from build123d import *

# Parameters (mm, degrees)
F0_W     = 36.068
F0_H     = 9.5504
F0_R     = 1.524
F0_H_2   = 16.9672
F0_W_2   = 16.002
F0_R_2   = 2.2225
F1_DEPTH = 1.7018
F2_R     = 2.54
F3_R     = 2.54
F4_W     = 5.766904
F4_H     = 5.702107
F5_DEPTH = 1.778


with BuildPart() as f1:
    # F0 (on Top) → F1 (new body)
    with BuildSketch(Plane.XY):
        with Locations((0, -13.2588)):
            Rectangle(F0_W, F0_H)
        with Locations((-15.167683, -15.197962)):
            Circle(F0_R, mode=Mode.SUBTRACT)
        with Locations((15.185317, -15.197962)):
            Circle(F0_R, mode=Mode.SUBTRACT)
        Rectangle(F0_W, F0_H_2)
        with Locations((-26.035, 0)):
            Rectangle(F0_W_2, F0_H_2)
        with Locations((-29.552327, -3.693333)):
            Circle(F0_R_2, mode=Mode.SUBTRACT)
        with Locations((-29.552327, 3.545667)):
            Circle(F0_R_2, mode=Mode.SUBTRACT)
        with Locations((0, 13.2588)):
            Rectangle(F0_W, F0_H)
        with Locations((-15.167683, 15.155038)):
            Circle(F0_R, mode=Mode.SUBTRACT)
        with Locations((15.185317, 15.155038)):
            Circle(F0_R, mode=Mode.SUBTRACT)
    extrude(amount=F1_DEPTH)

    # F2
    f2_edges = [f1.edges().sort_by_distance(p)[0] for p in [
        (-18.034, 18.034, 0.8509),
        (-18.034, -18.034, 0.8509),
        (18.034, -18.034, 0.8509),
        (18.034, 18.034, 0.8509),
    ]]
    fillet(f2_edges, radius=F2_R)

    # F3
    f3_edges = [f1.edges().sort_by_distance(p)[0] for p in [
        (-18.034, 8.4836, 0.8509),
        (-18.034, -8.4836, 0.8509),
        (-34.036, -8.4836, 0.8509),
        (-34.036, 8.4836, 0.8509),
    ]]
    fillet(f3_edges, radius=F3_R)

    # F4 (on face) → F5 (join)
    with BuildSketch(Plane.XY.offset(1.7018)):
        with Locations((-4.934564, 7.768857)):
            Rectangle(F4_W, F4_H)
    extrude(amount=F5_DEPTH)


solid = f1.part
Read the model definition and answer for the solid it produces. Units are mm, in the model's axes. A direction names the side the tool comes from. Give positions to 0.01 mm unless a question says otherwise; leave off trailing zeros. Write each loop counter-clockwise with the first axis right and the second up, starting at its lowest first coordinate (ties: lowest second). Pieces come first, ordered by that corner, then holes. Notation, with made-up numbers: M 66.25,29 L 102.25,29 A20 cw 102.25,51 Z; hole C -37,10 d6. An arc over 180 degrees is marked long. One line per item, written item: value. Start each with the question number.
(1) Find section A-A (x = -3). Determine the outline of the cut face in (y, z).
(2) Find section D-D (z = 1.1). Determine the outline of the cut face in (x, y) (1 decimal), plus the area to 3 significant figures.
(3) Flat-ended cylindrical pins translate along their axes: pin 1 Ø5 at (x, y) = (-9.5, 11) entering from -Z; pin 2 Ø0.5 at (y, z) = (7.5, 2.5) entering from +X; pin 3 Ø1.4 at (y, z) = (14, 0.5) entering from -X; pin 4 Ø2.5 at (x, y) = (15.19, 15.16) entering from +Z. Find the tip coordinate at first contact, or state that the pin passes through.
(4) A tool of negligible diameter and unlimited length cuts with its end or side. For faces 4 (the cylindrical face through (-27.43, -3.03, 0.84)), 5 (the flat face through (-2.051, 8, 3)), 6 (the flat face through (-5, 10.62, 3)), 7 (the flat face through (-18.034, 13, 1)), 8 (the flat face through (-18.034, -13, 1)), from which of +Z, -Z, +X, -X, +Y, -Y can it reach the whole face along a straight path? Write none if from no direction.
(5) Find section C-C (x = -14.5). Determine the outline of the cut face in (y, z) (3 decimals), plus the area to 3 significant figures.
(6) Find the intervals of material crossed by line 1 (X direction, y = -14, z = 1.25); line 2 (X direction, y = 16, z = 1.3); line 3 (Z direction, x = 7, y = -16), in increasing order.
(7) Determine the mould class of faces 1 (the flat face through (-34.036, 0, 1)), 2 (the flat face through (0, 18.034, 1)), 3 (the cylindrical face through (-27.43, 4.21, 0.84)) for opening direction X: pulls with the +X half, pulls with the -X half, needs draft (parallel to the pull), parting line crosses it, or undercut.
(8) Find section B-B (y = 2). Determine the outline of the cut face in (x, z).
Results below:
1. outline: M -18.03,0 L 18.03,0 L 18.03,1.7 L 10.62,1.7 L 10.62,3.48 L 4.92,3.48 L 4.92,1.7 L -18.03,1.7 Z
2. outline: M -34,-5.9 A2.5 ccw -31.5,-8.5 L -20.6,-8.5 A2.5 cw -18,-11 L -18,-15.5 A2.5 ccw -15.5,-18 L 15.5,-18 A2.5 ccw 18,-15.5 L 18,15.5 A2.5 ccw 15.5,18 L -15.5,18 A2.5 ccw -18,15.5 L -18,11 A2.5 cw -20.6,8.5 L -31.5,8.5 A2.5 ccw -34,5.9 Z; hole C -29.6,-3.7 d4.4; hole C -29.6,3.5 d4.4; hole C -15.2,-15.2 d3; hole C -15.2,15.2 d3; hole C 15.2,-15.2 d3; hole C 15.2,15.2 d3
2. area: 1,510 mm^2
3. pin 1: stops at z = 0
3. pin 2: stops at x = -2.05
3. pin 3: stops at x = -18.03
3. pin 4: passes through
4. face 4: +Z, -Z
4. face 5: +Z, +X, +Y, -Y
4. face 6: +Z, +X, -X, +Y
4. face 7: +Z, -Z, -X, +Y
4. face 8: +Z, -Z, -X, -Y
5. outline: M -18.034,0 L -16.568,0 L -16.568,1.702 L -18.034,1.702 Z; M -13.828,0 L 13.785,0 L 13.785,1.702 L -13.828,1.702 Z; M 16.525,0 L 18.034,0 L 18.034,1.702 L 16.525,1.702 Z
5. area: 52.1 mm^2
6. line 1: x = -18.03 to -16.11, -14.23 to 14.24, 16.13 to 18.03
6. line 2: x = -17.98 to -16.44, -13.9 to 13.92, 16.45 to 17.98
6. line 3: z = 0 to 1.7
7. face 1: pulls with the -X half
7. face 2: needs draft
7. face 3: undercut
8. outline: M -34.04,0 L -31.15,0 L -31.15,1.7 L -34.04,1.7 Z; M -27.96,0 L 18.03,0 L 18.03,1.7 L -27.96,1.7 Z
